For this review, take the finished solid that the model builds, in its own axes (mm). Face numbers are marked on the shaded views. A direction names the side the tool comes from. Coordinates: 2 decimals unless noted, no trailing zeros. Write each loop counter-clockwise with the first axis right and the second up, starting at its lowest first coordinate (ties: lowest second). Pieces come first, ordered by that corner, then holes.
1) For the marked faces 1 and 2, list the 3-axis set-ups (+Z, -Z, +X, -X, +Y, -Y) from which the entire face can be reached by the end or side of a thin tool; tool diameter is ignored.
2) We need section B-B on x = 20. Write out the cut boundary in (y, z), then the cut area to 3 significant figures.
3) To check wall thickness, follow line 1 along Z through (x, y) = (-19, 0); line 2 along Z through (x, y) = (-20.25, 0); line 3 along Y through (x, z) = (-29, 0.75). State the ranges of each line that lie inside material, in increasing order.
4) Insertion check: P1, Ø2, axis at x = -10, y = -2.5, coming from the +Z side; P2, Ø2, axis at x = 1.5, z = 2, coming from the +Y side; P3, Ø1.5, axis at x = 24, y = 5, coming from the -Z side. Each pin has a flat end and moves straight along its axis. Give the tip position at first contact, or say it passes through.
5) We need section A-A on x = -14.5. Write out the cut boundary in (y, z), then the cut area to 3 significant figures.
from build123d import *

# Parameters (mm, degrees)
F2_R     = 9.398
F4_R     = 7.62
F5_R     = 0.9906
F6_DEPTH = 25.4


# Not quite as in the source:
# - a fillet or chamfer that OpenCascade refuses, or shapes differently, is made with other operations: its cross-section is extruded or revolved along the edge and cut away or added


with BuildPart() as f1:
    # F0 (on Front) → F1 (revolve)
    with BuildSketch(Plane.XZ):
        Polygon((-32.9808058875, 0), (0, 0), (31.0198143902, 0), (31.0271941125, 9.4996), (-24.9798058875, 9.4996), (-24.9798058875, 4.2418), (-32.9808058875, 4.2418), align=None)
    revolve(axis=Axis((15.5099071951, 0, 0), (1, 0, 0)))

    # F2
    f2_edges = [f1.edges().sort_by_distance(p)[0] for p in [
        (31.027194, 0, -9.4996),
        (31.023504, 0, 4.7498),
    ]]
    fillet(f2_edges, radius=F2_R)

    # F3: fillet of radius 9.398 on 1 edges, made by hand

    # F3_s1 → F3_t2 (revolve, cut)
    with BuildSketch(Plane.XZ):
        with BuildLine():
            ThreePointArc((-16.542913808, 9.4996), (-21.5134673185, 8.0775640044), (-24.9798058875, 4.2418))
            Line((-24.9798058875, 4.2418), (-24.9798058875, 9.4996))
            Line((-24.9798058875, 9.4996), (-16.542913808, 9.4996))
        make_face()
    revolve(axis=Axis((-24.9798058875, 0, 0), (1, 0, 0)), mode=Mode.SUBTRACT)

    # F4
    f4_edges = [f1.edges().sort_by_distance(p)[0] for p in [
        (-24.979806, 0, -4.2418),
    ]]
    fillet(f4_edges, radius=F4_R)

    # F5 (on face) → F6 (cut)
    with BuildSketch(Plane(origin=(-32.9808058875, 0, 0), x_dir=(0, -1, 0), z_dir=(-1, 0, 0))):
        Circle(F5_R)
    extrude(amount=-F6_DEPTH, mode=Mode.SUBTRACT)


solid = f1.part
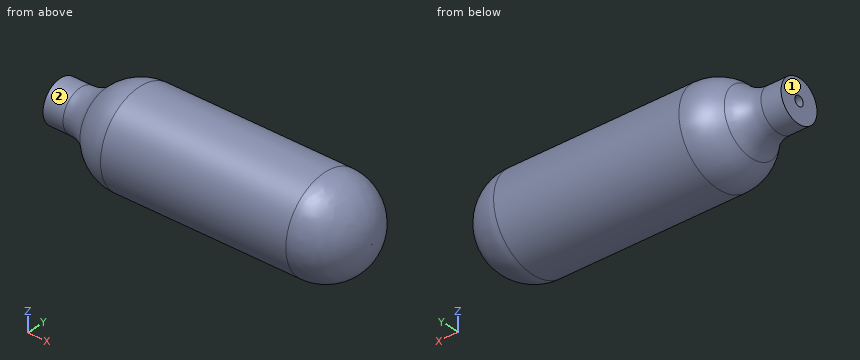
Result:
1. face 1: +Z, -Z, -X, +Y, -Y
1. face 2: -X
2. outline: circle Ø19 at (0, 0)
2. area: 284 mm2
3. line 1: z = -9.17 to -0.99, 0.99 to 9.17
3. line 2: z = -8.74 to -0.99, 0.99 to 8.74
3. line 3: y = -4.17 to -0.65, 0.65 to 4.17
4. P1: stops at z = 9.38
4. P2: stops at y = 9.45
4. P3: stops at z = -8.2
5. outline: circle Ø19 at (0, 0); hole circle Ø1.98 at (0, 0)
5. area: 280 mm2
